Read the model definition and answer for the solid it produces. Units are mm, in the model's axes. Face numbers are marked on the shaded views. Give positions to 0.01 mm unless a question says otherwise; leave off trailing zeros. Order: outer loops, then holes, each group sorted by start corner. A loop starts at its lowest first (then second) coordinate and runs counter-clockwise, first axis right, second up. Notation, with made-up numbers: (-26, 43) -> (16, 43) arc R28 cw to (16, 81) -> close; hole circle Ø10 at (69, -26.5). An arc over 180 degrees is marked (long way). One line per item, written item: value. Start each with the question number.
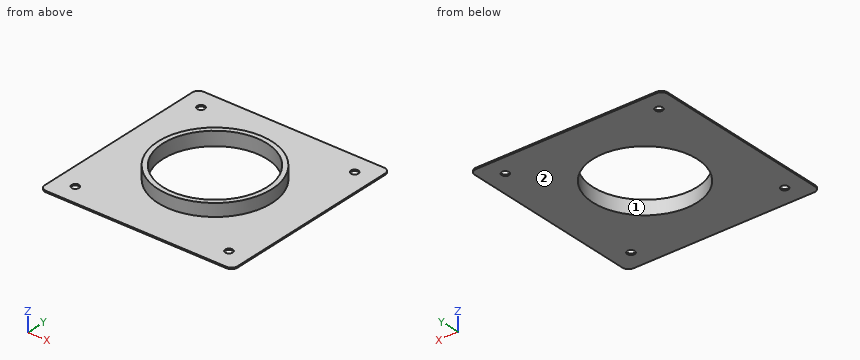
Autodesk Inventor part; units mm, degrees
ref_plane "YZ Plane" through (0, 0, 0) normal (1, 0, 0) x (0, 1, 0)
ref_plane "XZ Plane" through (0, 0, 0) normal (0, 1, 0) x (-1, 0, 0)
ref_plane "XY Plane" through (0, 0, 0) normal (0, 0, 1) x (1, 0, 0)
sketch "Sketch1" plane through (0, 0, 0) normal (0, 0, 1) x (1, 0, 0)
  line L0 (-25.4072, 25.3665) -> (76.1928, 25.3665)
  line L1 (76.1928, 25.3665) -> (76.1928, -76.2335)
  line L2 (76.1928, -76.2335) -> (-25.4072, -76.2335)
  line L3 (-25.4072, -76.2335) -> (-25.4072, 25.3665)
  point P0 (0, 0)
  dimension "d0" = 101.6
  dimension "d1" = 101.6
extrude "Extrusion1" add sketch "Sketch1" along normal blind 0.7366
sketch "Sketch2" plane through (0, 0, 0.7366) normal (0, 0, 1) x (1, 0, 0)
  line L0 (-25.4072, 25.3665) -> (76.1928, -76.2335)
  line L1 (76.1928, 25.3665) -> (-25.4072, -76.2335)
  circle A0 centre (25.3928, -25.4335) radius 27.432
  point P0 (0, 0)
  dimension "d4" = 54.864
extrude "Extrusion2" cut sketch "Sketch2" against normal blind 0.7366
sketch "Sketch3" plane through (0, 0, 0.7366) normal (0, 0, 1) x (1, 0, 0)
  line L0 (-25.4072, -76.2335) -> (-25.4072, 25.3665)
  line L1 (-25.4072, 25.3665) -> (-25.4072, -25.4335)
  line L2 (-25.4072, -25.4335) -> (-25.4072, 19.4102)
  line L3 (-25.4072, 25.3665) -> (76.1928, -76.2335)
  line L4 (76.1928, 25.3665) -> (-25.4072, -76.2335)
  circle A0 centre (-19.4509, 19.4102) radius 1.9812
  point P0 (0, 0)
  dimension "d7" = 44.8437
  dimension "d8" = 3.9624
extrude "Extrusion3" cut sketch "Sketch3" against normal blind 0.7366 contours A0 L3 | L3 A0
sketch "Sketch4" plane through (0, 0, 0.7366) normal (0, 0, 1) x (1, 0, 0)
  line L0 (-25.4072, -76.2335) -> (76.1928, 25.3665)
  line L1 (-25.4072, 25.3665) -> (76.1928, -76.2335)
  circle A0 centre (70.2365, 19.4102) radius 1.9819
  circle A1 centre (70.2365, -70.2772) radius 1.983
  circle A2 centre (-19.4509, -70.2772) radius 1.9812
  point P0 (0, 0)
extrude "Extrusion4" cut sketch "Sketch4" against normal blind 0.7366
sketch "Sketch5" plane through (0, 0, 0.7366) normal (0, 0, 1) x (1, 0, 0)
  circle A0 centre (25.3928, -25.4335) radius 27.432
  circle A1 centre (25.3928, -25.4335) radius 29.972
  circle A2 centre (25.3928, -25.4335) radius 32.512
  point P0 (0, 0)
  dimension "d13" = 59.944
  dimension "d14" = 65.024
extrude "Extrusion5" add sketch "Sketch5" along normal blind 6.6548 contours A2
fillet "Fillet1" radius 3.175 4 edges at (-25.4072, 25.3665, 0.3683) (76.1928, 25.3665, 0.3683) (76.1928, -76.2335, 0.3683) (-25.4072, -76.2335, 0.3683)
sketch "Sketch6" plane through (25.3928, -25.4335, 0.7366) normal (0, 0, 1) x (1, 0, 0)
  circle A0 centre (0, 0) radius 29.972
  circle A1 centre (0, 0) radius 27.432
  point P0 (-25.3928, 25.4335)
extrude "Extrusion6" add sketch "Sketch6" along normal blind 9.1948
sketch "Sketch7" plane through (25.3928, -25.4335, 7.3914) normal (0, 0, 1) x (1, 0, 0)
  circle A0 centre (0, 0) radius 29.972
  circle A1 centre (0, 0) radius 32.512
  point P0 (-25.3928, 25.4335)
extrude "Extrusion7" cut sketch "Sketch7" against normal blind 6.6548
sketch "Sketch8" plane through (25.3928, -25.4335, 9.9314) normal (0, 0, 1) x (1, 0, 0)
  circle A0 centre (0, 0) radius 27.432
  circle A1 centre (0, 0) radius 29.972
  point P0 (-25.3928, 25.4335)
extrude "Extrusion8" cut sketch "Sketch8" against normal blind 2.54
sketch "Sketch9" plane through (0, 0, 0.7366) normal (0, 0, 1) x (1, 0, 0)
  circle A0 centre (-19.4509, 19.4102) radius 1.9812
  circle A1 centre (70.2365, -70.2772) radius 1.983
  circle A2 centre (-19.4509, -70.2772) radius 1.9812
  circle A3 centre (70.2365, 19.4102) radius 1.9819
  point P0 (0, 0)
extrude "Extrusion9" add sketch "Sketch9" against normal blind 0.7366
sketch "Sketch10" plane through (0, 0, 0.7366) normal (0, 0, 1) x (1, 0, 0)
  line L0 (-25.4072, 25.3665) -> (76.1928, 25.3665)
  line L1 (76.1928, 25.3665) -> (76.1928, -76.2335)
  line L2 (76.1928, -76.2335) -> (-25.4072, -76.2335)
  line L3 (-25.4072, -76.2335) -> (-25.4072, 25.3665)
  line L4 (-25.4072, 25.3665) -> (76.1928, -76.2335)
  line L5 (-25.4072, -76.2335) -> (76.1928, 25.3665)
  line L6 (-25.4072, 25.3665) -> (-25.4072, -25.4335)
  line L7 (-25.4072, -25.4335) -> (-25.4072, 15.0541)
  circle A0 centre (-15.0948, 15.0541) radius 1.9812
  circle A1 centre (65.8804, 15.0541) radius 1.9818
  circle A2 centre (65.8804, -65.9211) radius 1.9832
  circle A3 centre (-15.0948, -65.9211) radius 1.9812
  point P0 (0, 0)
  dimension "d26" = 40.4876
  dimension "d27" = 3.9624
extrude "Extrusion10" cut sketch "Sketch10" against normal blind 0.7366 contours A0 L4 | L4 A0 | A1 L5 | L5 A1 | A2 L4 | L4 A2 | A3 L5 | L5 A3
properties part number "2"
Item 1: Find section B-B on y = -49. Write down the section's boundary in (x, z), then the cut area to 3 significant figures.
Item 2: Find the intervals of material crossed by line 1 (Z direction, x = 53.5, y = -54); line 2 (X direction, y = -46, z = 5); line 3 (X direction, y = -7, z = 6.5), in increasing order. Write a range as from..to.
Item 3: For a pull along Y with two mould halves and no side action, classify the marked faces 1 and 2 as +Y half, -Y half, draft (parallel to the pull), parting line (faces both ways), or undercut.
Item 4: Find section C-C on z = 3.5. Write down the section's boundary in (x, y).
Item 5: Find section A-A on x = 8.5. Write down the section's boundary in (y, z).
Item 6: Flat-ended cylindrical pins translate along their axes: pin 1 (6.5 mm diameter, centred on x = 65.88, y = 15.05, fed in from +Z); pin 2 (2.5 mm diameter, centred on x = -15.09, y = 15.05, fed in from -Z). Find the tip coordinate at first contact, or state that the pin passes through.
Item 7: Find section D-D on y = -61.5. Write down the section's boundary in (x, z), then the cut area to 3 significant figures.
Checks:
1. outline: (-25.41, 0) -> (11.35, 0) -> (11.35, 7.39) -> (6.87, 7.39) -> (6.87, 0.74) -> (-25.41, 0.74) -> close; (39.43, 0) -> (76.19, 0) -> (76.19, 0.74) -> (43.91, 0.74) -> (43.91, 7.39) -> (39.43, 7.39) -> close
1. area: 114 mm2
2. line 1: 0..0.74
2. line 2: 3.59..7.24, 43.55..47.2
2. line 3: 1.76..5.08, 45.71..49.03
3. face 1: undercut
3. face 2: draft
4. outline: circle Ø59.94 at (25.39, -25.43); hole circle Ø54.86 at (25.39, -25.43)
5. outline: (-76.23, 0) -> (-47.05, 0) -> (-47.05, 7.39) -> (-50.19, 7.39) -> (-50.19, 0.74) -> (-76.23, 0.74) -> close; (-3.82, 0) -> (25.37, 0) -> (25.37, 0.74) -> (-0.68, 0.74) -> (-0.68, 7.39) -> (-3.82, 7.39) -> close
6. pin 1: z = 0.74
6. pin 2: through
7. outline: (-25.41, 0) -> (76.19, 0) -> (76.19, 0.74) -> (-25.41, 0.74) -> close
7. area: 74.8 mm2
